Input: dimensioned drawing with shaded views. Units: mm. Origin: part minimum x, y, z. Give positions to 0.01 mm unless a question says otherwise; leave off trailing zeros. Write each loop counter-clockwise with the first axis right and the second up, starting at its lowest first coordinate (ties: lowest second). Pieces come first, ordered by that corner, then holes. Notation, with made-up numbers: (73, -23.5) -> (88, -23.5) arc R12 ccw to (88, -8.5) -> close; hole circle Ø7 at (45.25, 85.5). An arc over 180 degrees is marked (long way). Return JSON: item names as keys, results as strings. Group by question number.
Item 1: Mould query, pull axis Z, two halves, no side actions, for the marked faces 1 and 2. Classes: released by +Z, released by -Z, zero draft, split by the parting line, or undercut.
Item 2: Line query: line 1 (X direction, y = 23.5, z = 23.5); line 2 (X direction, y = 18, z = 14.75); line 3 (Z direction, x = 96.5, y = 16). Output: solid intervals per line, ascending. Write a range as [from, to].
Item 3: Pin query (flat end, axial travel): P1, Ø8, axis at x = 310, z = 19.5, coming from the -Y side; P2, Ø5, axis at y = 22.5, z = 7.5, coming from the +X side; P3, Ø12, axis at x = 140, z = 6.5, coming from the +Y side. Return the tip coordinate at first contact, or that it passes through.
Item 4: Section A-A, the plane x = 154. Return loops of the section in (y, z), then the cut area to 3 significant figures.
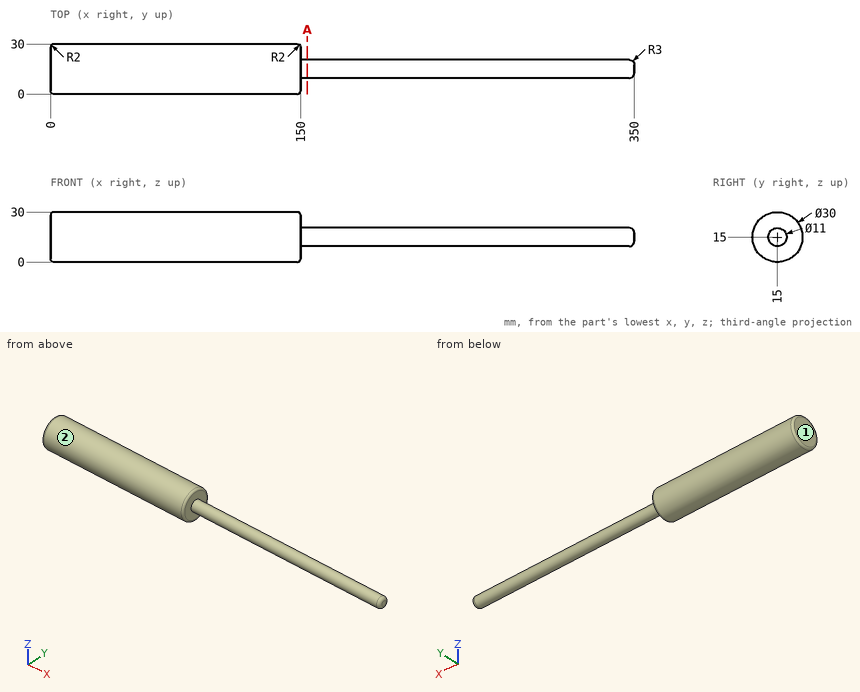
Answer below:
{
 "1": {"face 1": "zero draft", "face 2": "split by the parting line"},
 "2": {"line 1": "x = [0, 150]", "line 2": "x = [0, 349.96]", "line 3": "z = [0.03, 29.97]"},
 "3": {"P1": "stops at y = 9.52", "P2": "stops at x = 150", "P3": "stops at y = 29.79"},
 "4": {"outline": "circle Ø11 at (15, 15)", "area": "95.0 mm2"}
}
